Input: dimensioned drawing with shaded views. Units: mm. Origin: part minimum x, y, z. A direction names the side the tool comes from. Round coordinates to 2 decimals unless told otherwise and drop trailing zeros. Loops run counter-clockwise (first coordinate to the right, second up) from the corner with the lowest first, then second, coordinate; pieces in that order, holes last. Notation, with made-up numbers: M 33,16.25 L 71,16.25 A17 cw 71,45.25 Z; hole C 22.25,48.25 d5. An arc over 180 degrees is marked long. Use one line per item in the form item = value. Start each with the question number.
Q1. Section query C-C, the plane z = 2.75. Output: boundary loops of the cut face in (x, y).
Q2. Ray query, line 1 along Y through (x, z) = (4.25, 1.5); line 2 along X through (y, z) = (12.25, 7.5). Return the intervals inside material, ascending.
Q3. Access query for the marked faces 5, 6 and 7. Directions: +Z, -Z, +X, -X, +Y, -Y. A direction counts if a zero-diameter tool reaches every point of the face in a straight line with its end or side. Return the directions, or none.
Q4. Section query D-D, the plane x = 10. Output: boundary loops of the cut face in (y, z).
Q5. Mould query, pull axis Z, two halves, no side actions, for the marked faces 1, 2, 3 and 4. Classes: pulls with the +Z half, pulls with the -Z half, needs draft (parallel to the pull), parting line crosses it, or undercut.
Q6. Section query A-A, the plane z = 5. Output: boundary loops of the cut face in (x, y), and give its area (3 significant figures).
Q7. First-contact query: P1, Ø8, axis at x = 16, z = 15, coming from the -Y side; P2, Ø1.5, axis at x = 14, y = 25, coming from the -Z side. Flat tips, straight axial feed; report the tip coordinate or a pass-through.
Q8. Section query B-B, the plane y = 5.75. Output: boundary loops of the cut face in (x, z).
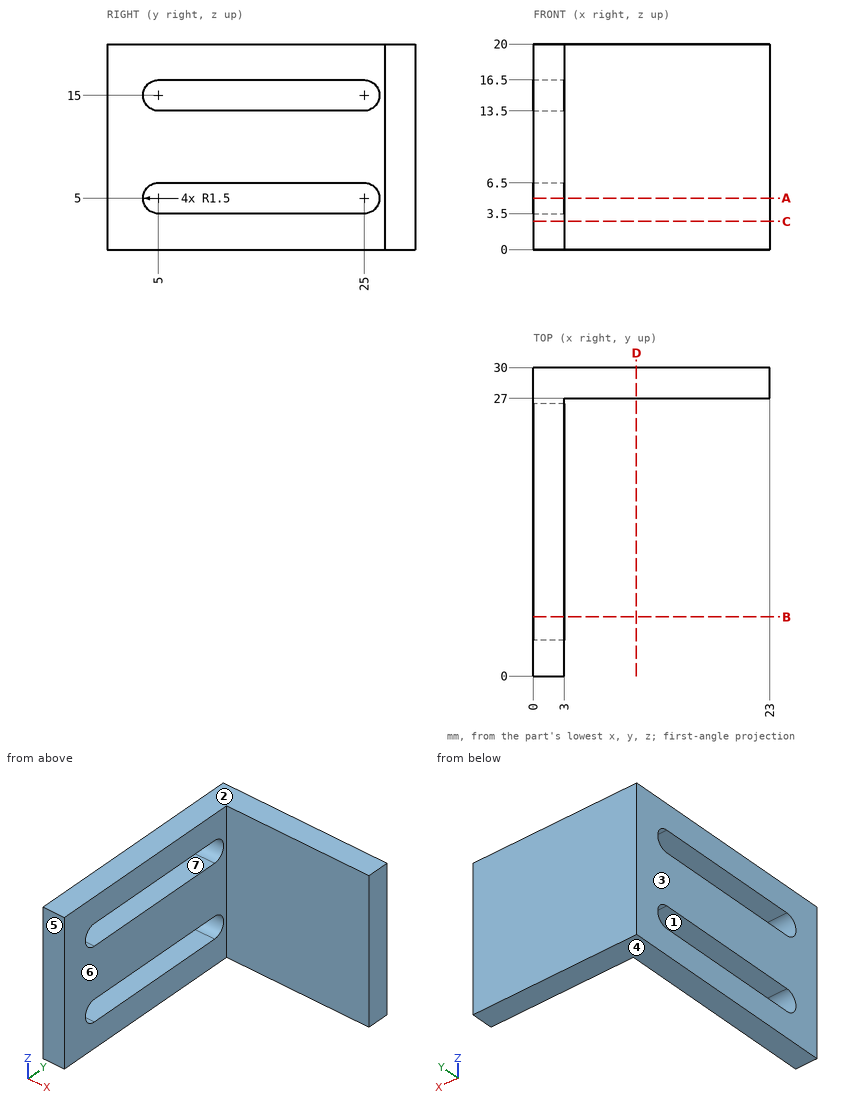
Results found:
q1.outline = M 0,0 L 3,0 L 3,27 L 23,27 L 23,30 L 0,30 Z
q2.line_1 = 27 to 30
q2.line_2 = 0 to 3
q3.face_5 = +Z, -Z, +X, -X, -Y
q3.face_6 = +Z, -Z, +X, -Y
q3.face_7 = +X, -X
q4.outline = M 27,0 L 30,0 L 30,20 L 27,20 Z
q5.face_1 = undercut
q5.face_2 = pulls with the +Z half
q5.face_3 = needs draft
q5.face_4 = pulls with the -Z half
q6.outline = M 0,0 L 3,0 L 3,3.5 L 0,3.5 Z; M 0,26.5 L 3,26.5 L 3,27 L 23,27 L 23,30 L 0,30 Z
q6.area = 81.0 mm²
q7.P1 = 27
q7.P2 = through
q8.outline = M 0,0 L 3,0 L 3,3.5 L 0,3.5 Z; M 0,6.5 L 3,6.5 L 3,13.5 L 0,13.5 Z; M 0,16.5 L 3,16.5 L 3,20 L 0,20 Z
